```python
from build123d import *

# Parameters (mm, degrees)
F1_DEPTH = 5


# Not quite as in the source:
# - a feature names something its author has since deleted; it is built from what else it names


with BuildPart() as f1:
    # F0 (on Top) → F1 (new body)
    with BuildSketch(Plane.XY):
        Polygon((-3.25, -21), (-21, -21), (-21, -26.5), (-21, -56.5), (-15.25, -56.5), (-15.25, -44.75), (-15.25, -38.25), (-15.25, -26.5), (-3.75, -26.5), (0, -26.5), (3.75, -26.5), (15.25, -26.5), (15.25, -38.25), (15.25, -44.75), (15.25, -56.5), (21, -56.5), (21, -26.5), (21, -21), (3.25, -21), (0, -21), align=None)
        Polygon((0, -26.5), (-3.75, -26.5), (-3.75, -29), (-10.875, -29), (-5.5, -33.75), (0, -33.75), (5.5, -33.75), (10.875, -29), (3.75, -29), (3.75, -26.5), align=None)
        Polygon((-15.25, -38.25), (-15.25, -44.75), (-12.5, -44.75), (-12.5, -51.875), (-7.75, -47), (-7.75, -41.5), (-7.75, -36), (-12.5, -31.125), (-12.5, -38.25), align=None)
        Polygon((12.5, -44.75), (15.25, -44.75), (15.25, -38.25), (12.5, -38.25), (12.5, -31.125), (7.75, -36), (7.75, -41.5), (7.75, -47), (12.5, -51.875), align=None)
    extrude(amount=F1_DEPTH)


solid = f1.part
```
Read the model definition and answer for the solid it produces. Units are mm, in the model's axes. A direction names the side the tool comes from. Give positions to 0.01 mm unless a question says otherwise; leave off trailing zeros. Order: outer loops, then holes, each group sorted by start corner. A loop starts at its lowest first (then second) coordinate and runs counter-clockwise, first axis right, second up. Notation, with made-up numbers: (-36.5, 27.25) -> (-17.5, 27.25) arc R30 cw to (-17.5, 66.25) -> close; hole circle Ø9 at (22, -26.5). An arc over 180 degrees is marked (long way). One line per item, written item: value. Start each with the question number.
(1) The part is cut by section B-B (x = -13.5). Determine the outline of the cut face in (y, z).
(2) The part is cut by section A-A (y = -42). Determine the outline of the cut face in (x, z).
(3) A tool of negligible diameter and unlimited length cuts with its end or side. For faces 4 (the flat face through (-15.25, -32, 2)), 5 (the flat face through (-10.158, -49.472, 2.465)), 6 (the flat face through (-18, -56.5, 2)), from which of +Z, -Z, +X, -X, +Y, -Y can it reach the whole face along a straight path? Write none if from no direction.
(4) Flat-ended cylindrical pins translate along their axes: P1, Ø1.5, axis at x = -9.5, z = 3.5, coming from the -Y side; P2, Ø3, axis at x = 1.5, z = 3.5, coming from the -Y side. Find the tip coordinate at first contact, or state that the pin passes through.
(5) For a pull along X with two mould halves and no side action, classify faces 1 (the flat face through (21, -39, 2)), 2 (the flat face through (14, -44.75, 2)), 3 (the flat face through (0, -31, 0)) as released by +X, released by -X, zero draft, split by the parting line, or undercut.
(6) Straight lines are drawn through the part: L1, parallel to X at y = -36, z = 4.5; L2, parallel to X at y = -39.5, z = 1.1; L3, parallel to X at y = -53.5, z = 2.85. For each, find the intervals that lie inside material, in ascending order.
(7) The part is cut by section C-C (y = -35.5). Determine the outline of the cut face in (x, z), and give its area (3 significant figures).
Taken from the geometry:
1. outline: (-44.75, 0) -> (-38.25, 0) -> (-38.25, 5) -> (-44.75, 5) -> close; (-26.5, 0) -> (-21, 0) -> (-21, 5) -> (-26.5, 5) -> close
2. outline: (-21, 0) -> (-7.75, 0) -> (-7.75, 5) -> (-21, 5) -> close; (7.75, 0) -> (21, 0) -> (21, 5) -> (7.75, 5) -> close
3. face 4: +Z, -Z
3. face 5: +Z, -Z, -Y
3. face 6: +Z, -Z, +X, -X, -Y
4. P1: y = -49.57
4. P2: y = -33.75
5. face 1: released by +X
5. face 2: undercut
5. face 3: zero draft
6. L1: -21 to -15.25, -12.5 to -7.75, 7.75 to 12.5, 15.25 to 21
6. L2: -21 to -7.75, 7.75 to 21
6. L3: -21 to -15.25, 15.25 to 21
7. outline: (-21, 0) -> (-15.25, 0) -> (-15.25, 5) -> (-21, 5) -> close; (-12.5, 0) -> (-8.24, 0) -> (-8.24, 5) -> (-12.5, 5) -> close; (8.24, 0) -> (12.5, 0) -> (12.5, 5) -> (8.24, 5) -> close; (15.25, 0) -> (21, 0) -> (21, 5) -> (15.25, 5) -> close
7. area: 100 mm^2
